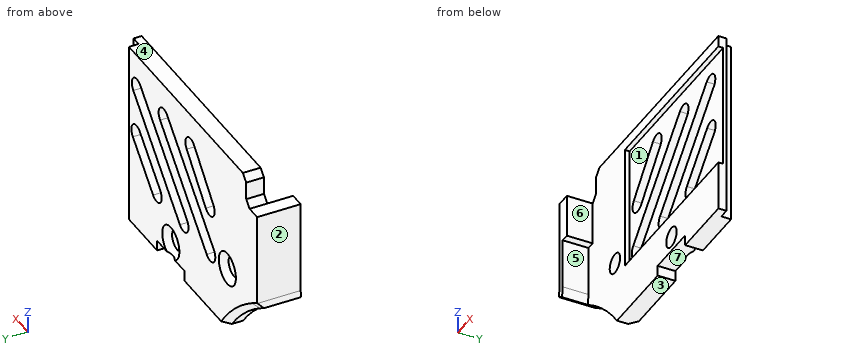
from build123d import *

# Parameters (mm, degrees)
SKETCH_221_R           = 1.55
EXTRUDE_926_DEPTH      = 2.75
SKETCH_1005_W          = 35.000000002
SKETCH_1005_H          = 4.75
EXTRUDE_1111_DEPTH     = 2.75
EXTRUDE_1_DEPTH        = 2.75
F_2_PCB_START          = -4
F_2_PCB_DEPTH          = 4
SKETCH_2154_W          = 1.5
SKETCH_2154_H          = 28.99988509
EXTRUDE_2226_DEPTH     = 1.25
SKETCH_2278_W          = 27.915979255
SKETCH_2278_H          = 19.5
PCB_DEPTH              = 0.75
CUT_EXTRUDE_2_DEPTH    = 33.451352798
CHAMFER_1_SIZE         = 1
CHAMFER_2_SIZE         = 1
CUT_EXTRUDE_3375_DEPTH = 4


with BuildPart() as part:
    # Sketch 221 → Extrude 926 (new body)
    with BuildSketch(Plane(origin=(0, 0, 0), x_dir=(1, 0, 0), z_dir=(0, 1, 0))):
        with BuildLine():
            ThreePointArc((-16.252981126, 10), (-20.15501929, 5.688743466), (-24.715186194, 2.08073674))
            Line((-24.715186194, 2.08073674), (-24.500000002, 0.312480077))
            Line((-24.500000002, 0.312480077), (-24.500000002, -7.263629174))
            Line((-24.500000002, -7.263629174), (-22.500000002, -7.263629174))
            Line((-22.500000002, -7.263629174), (-22.500000002, -14.24988509))
            Line((-22.500000002, -14.24988509), (12.5, -14.24988509))
            Line((12.5, -14.24988509), (12.5, 10))
            Line((12.5, 10), (4.100927374, 10))
            Line((4.100927374, 10), (4.100927374, 8.35804307))
            Line((4.100927374, 8.35804307), (-4.100927378, 8.35804307))
            Line((-4.100927378, 8.35804307), (-4.100927378, 10))
            Line((-4.100927378, 10), (-16.252981126, 10))
        make_face()
        with Locations(Location((-16.865979255, 0, 0), (0, 0, 270))):
            Circle(SKETCH_221_R, mode=Mode.SUBTRACT)
        with Locations(Location((-2e-09, 6.108043073, 0), (0, 0, 270))):
            Circle(SKETCH_221_R, mode=Mode.SUBTRACT)
    extrude(amount=EXTRUDE_926_DEPTH)

    # Sketch 1005 → Extrude 1111 (add)
    with BuildSketch(Plane(origin=(0, 0, 0), x_dir=(1, 0, 0), z_dir=(0, 1, 0))):
        with Locations((-5.000000001, -16.62488509)):
            Rectangle(SKETCH_1005_W, SKETCH_1005_H)
    extrude(amount=EXTRUDE_1111_DEPTH)

    # Sketch 1191 → 卡榫结构-1 (add)
    with BuildSketch(Plane(origin=(0, 0, 0), x_dir=(1, 0, 0), z_dir=(0, 1, 0))):
        with BuildLine():
            Line((-25.750000002, -14.213629174), (-22.500000002, -14.213629174))
            Line((-22.500000002, -14.213629174), (-22.500000002, -7.263629174))
            Line((-22.500000002, -7.263629174), (-24.500000002, -7.263629174))
            Line((-24.500000002, -7.263629174), (-24.500000002, 0.312480077))
            Line((-24.500000002, 0.312480077), (-24.715186194, 2.08073674))
            ThreePointArc((-24.715186194, 2.08073674), (-25.291636518, 1.705823535), (-25.875319612, 1.342273079))
            Line((-25.875319612, 1.342273079), (-25.750000002, 0.312480077))
            Line((-25.750000002, 0.312480077), (-25.750000002, -14.213629174))
        make_face()
    extrude(amount=EXTRUDE_1_DEPTH)

    # 草图5<4> → 卡榫结构-2-注意PCB凸出部分 (add)
    with BuildSketch(Plane(origin=(0, 0, 0), x_dir=(1, 0, 0), z_dir=(0, 1, 0)).offset(F_2_PCB_START)):
        with BuildLine():
            Line((-25.750000002, -14.213629174), (-23.500000002, -14.213629174))
            Line((-23.500000002, -14.213629174), (-23.500000002, -7.263629174))
            Line((-23.500000002, -7.263629174), (-24.500000002, -7.263629174))
            Line((-24.500000002, -7.263629174), (-24.500000002, 0.312480077))
            Line((-24.500000002, 0.312480077), (-24.715186194, 2.08073674))
            ThreePointArc((-24.715186194, 2.08073674), (-25.291636518, 1.705823535), (-25.875319612, 1.342273079))
            Line((-25.875319612, 1.342273079), (-25.750000002, 0.312480077))
            Line((-25.750000002, 0.312480077), (-25.750000002, -14.213629174))
        make_face()
    extrude(amount=F_2_PCB_DEPTH)

    # Sketch 2154 → Extrude 2226 (add)
    with BuildSketch(Plane(origin=(0, 0, 0), x_dir=(1, 0, 0), z_dir=(0, 1, 0))):
        with Locations((13.25, -4.499942545)):
            Rectangle(SKETCH_2154_W, SKETCH_2154_H)
    extrude(amount=EXTRUDE_2226_DEPTH)

    # Sketch 2278 → 稳压PCB器件高度补偿 (cut)
    with BuildSketch(Plane(origin=(0, 0, 0), x_dir=(1, 0, 0), z_dir=(0, 1, 0))):
        with Locations((0.042010372, -7.5)):
            Rectangle(SKETCH_2278_W, SKETCH_2278_H)
    extrude(amount=PCB_DEPTH, mode=Mode.SUBTRACT)

    # Sketch 2514 → 切除-拉伸2 (cut, through all)
    with BuildSketch(Plane.XZ.offset(-0.75)):
        with BuildLine():
            Line((3.173198201, 0.69066828), (9.20694903, 6.724419109))
            ThreePointArc((9.20694903, 6.724419109), (11.328269373, 6.724419109), (11.328269373, 4.603098766))
            Line((11.328269373, 4.603098766), (5.294518544, -1.430652063))
            ThreePointArc((5.294518544, -1.430652063), (3.173198201, -1.430652063), (3.173198201, 0.69066828))
        make_face()
        with BuildLine():
            Line((-4.826801799, 0.69066828), (9.08250112, 14.5999712))
            ThreePointArc((9.08250112, 14.5999712), (11.203821464, 14.5999712), (11.203821464, 12.478650856))
            Line((11.203821464, 12.478650856), (-2.705481456, -1.430652063))
            ThreePointArc((-2.705481456, -1.430652063), (-4.826801799, -1.430652063), (-4.826801799, 0.69066828))
        make_face()
        with BuildLine():
            Line((-12.826801799, 0.69066828), (1.08250112, 14.5999712))
            ThreePointArc((1.08250112, 14.5999712), (3.203821464, 14.5999712), (3.203821464, 12.478650856))
            Line((3.203821464, 12.478650856), (-10.705481456, -1.430652063))
            ThreePointArc((-10.705481456, -1.430652063), (-12.826801799, -1.430652063), (-12.826801799, 0.69066828))
        make_face()
        with BuildLine():
            Line((-4.738916917, 12.539185601), (-10.437516852, 6.169395501))
            ThreePointArc((-10.437516852, 6.169395501), (-12.555564069, 6.051599138), (-12.673360433, 8.169646355))
            Line((-12.673360433, 8.169646355), (-6.974760498, 14.539436455))
            ThreePointArc((-6.974760498, 14.539436455), (-4.856713281, 14.657232819), (-4.738916917, 12.539185601))
        make_face()
    extrude(amount=-CUT_EXTRUDE_2_DEPTH, mode=Mode.SUBTRACT)

    # 倒角1
    chamfer_1_edges = [part.edges().sort_by_distance(p)[0] for p in [
        (-20.661675073, 2.75, -5.223818951),
        (-22.500000002, 1.375, 18.99988509),
        (-22.500000002, 1.375, 14.213629174),
    ]]
    chamfer(chamfer_1_edges, length=CHAMFER_1_SIZE)

    # 倒角2
    # the kernel refuses this chamfer: 1 mm, written as the material it takes off along each edge
    with BuildSketch(Plane(origin=(-2e-09, 2.75, -6.108043073), x_dir=(0, 0, 1), z_dir=(-1, 0, 0))) as chamfer_2_piece_1:
        Polygon((1.55 + CHAMFER_2_SIZE, 0), (1.55, -CHAMFER_2_SIZE), (1.55, 0), align=None)
    revolve(axis=Axis((-2e-09, 2.75, -6.108043073), (0, 1, 0)), mode=Mode.SUBTRACT)
    with BuildSketch(Plane(origin=(-16.865979255, 2.75, 0), x_dir=(0, 0, 1), z_dir=(-1, 0, 0))) as chamfer_2_piece_2:
        Polygon((1.55 + CHAMFER_2_SIZE, 0), (1.55, -CHAMFER_2_SIZE), (1.55, 0), align=None)
    revolve(axis=Axis((-16.865979255, 2.75, 0), (0, 1, 0)), mode=Mode.SUBTRACT)

    # 草图1 → Cut-Extrude 3375 (cut)
    with BuildSketch(Plane.XZ.offset(4)):
        with BuildLine():
            Line((-24.715186194, -2.08073674), (-24.500000002, -0.312480077))
            Line((-24.500000002, -0.312480077), (-24.500000002, 7.263629174))
            Line((-24.500000002, 7.263629174), (-23.500000002, 7.263629174))
            Line((-23.500000002, 7.263629174), (-23.500000002, 7.513629174))
            Line((-23.500000002, 7.513629174), (-24.750000002, 7.513629174))
            Line((-24.750000002, 7.513629174), (-24.750000002, -0.312480077))
            Line((-24.750000002, -0.312480077), (-24.946632534, -1.928275128))
            ThreePointArc((-24.946632534, -1.928275128), (-24.830758909, -2.004277534), (-24.715186194, -2.08073674))
        make_face()
    extrude(amount=-CUT_EXTRUDE_3375_DEPTH, mode=Mode.SUBTRACT)


solid = part.part
Read the model definition and answer for the solid it produces. Units are mm, in the model's axes. Face numbers are marked on the shaded views. A direction names the side the tool comes from. Give positions to 0.01 mm unless a question says otherwise; leave off trailing zeros. Write each loop counter-clockwise with the first axis right and the second up, starting at its lowest first coordinate (ties: lowest second). Pieces come first, ordered by that corner, then holes. Notation, with made-up numbers: (-1.5, -17.75) - (55.5, -17.75) arc R28 ccw to (55.5, 21.25) - close; hole circle Ø2 at (-18.5, 34). An arc over 180 degrees is marked (long way). Return JSON: item names as keys, results as strings.
Q1. A cutting plane is placed at C-C, the plane y = -0.5. Determine the outline of the cut face in (x, z).
Reply:
{"outline": "(-25.88, -1.34) arc R35.11 cw to (-24.95, -1.93) - (-24.75, -0.31) - (-24.75, 7.51) - (-23.5, 7.51) - (-23.5, 14.21) - (-25.75, 14.21) - (-25.75, -0.31) - close"}
Q2. A cutting plane is placed at D-D, the plane y = 2.25. Count the separate pieces of the cut face and the enclosed holes in it, and give its area (3 significant figures).
Reply:
{"separate pieces": "1", "enclosed holes": "6", "area": "804 mm²"}
Q3. Given P1, Ø6, axis at x = 9, z = 7, coming from the -Y side; P2, Ø0.5, axis at y = 2, z = -9, coming from the -X side; P3, Ø12, axis at x = -10, z = 13, coming from the -Y side; P4, Ø2.5, axis at x = 0, z = -6.11, coming from the +Y side, each flat-ended and moving along its own axis, determine where each tip first touches the part or whether it passes through.
Reply:
{"P1": "y = 0.75", "P2": "x = -17.11", "P3": "y = 0", "P4": "through"}
Q4. Consider line 1 along Z through (x, y) = (0, 0.4); line 2 along X through (y, z) = (0.4, 0); line 3 along Z through (x, y) = (10, 2). Determine where each line is inside the solid, lowest interval first. Write a range as [from, to].
Reply:
{"line 1": "[-8.36, -7.66], [-4.56, -2.25], [17.25, 19]", "line 2": "[-25.75, -18.42], [-15.32, -13.92]", "line 3": "[-10, 3.27], [7.14, 11.27], [15.03, 19]"}
Q5. A cutting plane is placed at B-B, the plane x = -9. Determine the outline of the cut face in (y, z).
Reply:
{"outline": "(0, -10) - (2.75, -10) - (2.75, 0.27) - (0.75, 0.27) - (0.75, -2.25) - (0, -2.25) - close; (0, 17.25) - (0.75, 17.25) - (0.75, 12.28) - (2.75, 12.28) - (2.75, 19) - (0, 19) - close; (0.75, 4.52) - (2.75, 4.52) - (2.75, 7.78) - (0.75, 7.78) - close"}
Q6. For the marked faces 5, 6 and 7, determine the directions among +Z, -Z, +X, -X, +Y, -Y from which every point of the face is accessible in a straight line to the end or side of a thin tool.
Reply:
{"face 5": "-Z, +X, -Y", "face 6": "+Z, -Z, +X, -Y", "face 7": "-Z, +Y, -Y"}
Q7. A cutting plane is placed at A-A, the plane z = 15.75. Determine the outline of the cut face in (x, y).
Reply:
{"outline": "(-22.5, 0) - (-13.92, 0) - (-13.92, 0.75) - (14, 0.75) - (14, 1.25) - (12.5, 1.25) - (12.5, 2.75) - (-22.5, 2.75) - close"}
Q8. For a pull along Z with two mould halves and no side action, classify the marked faces 1, 2, 3 and 4 as released by +Z, released by -Z, zero draft, split by the parting line, or undercut.
Reply:
{"face 1": "undercut", "face 2": "zero draft", "face 3": "released by -Z", "face 4": "released by +Z"}
